Geometry check sheet. Reference: the model listing, model coordinates, mm. Face numbers are marked on the shaded views. Coordinates: 2 decimals unless noted, no trailing zeros. Loops run counter-clockwise (first coordinate to the right, second up) from the corner with the lowest first, then second, coordinate; pieces in that order, holes last.
from build123d import *

# Parameters (mm, degrees)
SKETCH1_W                            = 90
SKETCH1_H                            = 120
BOSS_EXTRUDE2_DEPTH                  = 4
SKETCH5_W                            = 12.2
SKETCH5_H                            = 22.5
CUT_EXTRUDE1_DEPTH                   = 76.106590923
BOSS_EXTRUDE4_START                  = 45
SKETCH10_W                           = 30.35
SKETCH10_H                           = 30.35
SKETCH10_R                           = 7.75
BOSS_EXTRUDE4_DEPTH                  = 25
BOSS_EXTRUDE5_START                  = -20
SKETCH10_4_W                         = 30.35
SKETCH10_4_H                         = 30.35
SKETCH10_4_R                         = 7.75
BOSS_EXTRUDE5_DEPTH                  = 25
CHAMFER6_SIZE                        = 5
CHAMFER7_SIZE                        = 10
F_3_0_3_DIAMETER_HOLE2_D             = 3
MIRROR9_AT_THE_SECOND_PLANE_COPY_1_D = 3
F_3_0_3_DIAMETER_HOLE3_D             = 3


with BuildPart() as part:
    # Sketch1 → Boss-Extrude2 (new body)
    with BuildSketch(Plane(origin=(0, 0, 0), x_dir=(1, 0, 0), z_dir=(0, 1, 0))):
        Rectangle(SKETCH1_W, SKETCH1_H)
    extrude(amount=BOSS_EXTRUDE2_DEPTH)

    # Sketch5 → Cut-Extrude1 (cut, through all)
    with BuildSketch(Plane(origin=(0, 4, 0), x_dir=(1, 0, 0), z_dir=(0, 1, 0))):
        with Locations((-23.9, 33.75)):
            Rectangle(SKETCH5_W, SKETCH5_H)
        with Locations((23.9, 33.75)):
            Rectangle(SKETCH5_W, SKETCH5_H)
    extrude(amount=-CUT_EXTRUDE1_DEPTH, mode=Mode.SUBTRACT)

    # Sketch10 → Boss-Extrude4 (add)
    # profile 1 of 3: a face of its own
    with BuildSketch(Plane(origin=(0, 0, 0), x_dir=(0, 0, -1), z_dir=(1, 0, 0)).offset(BOSS_EXTRUDE4_START)):
        with Locations((-29.825, 19.175)):
            Rectangle(SKETCH10_W, SKETCH10_H)
        with Locations((-29.825, 19.175)):
            Circle(SKETCH10_R, mode=Mode.SUBTRACT)
    # profile 2 of 3: a face of its own
    with BuildSketch(Plane(origin=(0, 0, 0), x_dir=(0, 0, -1), z_dir=(1, 0, 0)).offset(BOSS_EXTRUDE4_START)):
        with BuildLine():
            ThreePointArc((-25.604514246, 25.675), (-29.825, 26.925), (-34.045485754, 25.675))
            Line((-34.045485754, 25.675), (-25.604514246, 25.675))
        make_face()
    # profile 3 of 3: a face of its own
    with BuildSketch(Plane(origin=(0, 0, 0), x_dir=(0, 0, -1), z_dir=(1, 0, 0)).offset(BOSS_EXTRUDE4_START)):
        with BuildLine():
            Line((-25.604514246, 12.675), (-34.045485754, 12.675))
            ThreePointArc((-34.045485754, 12.675), (-29.825, 11.425), (-25.604514246, 12.675))
        make_face()
    extrude(amount=-BOSS_EXTRUDE4_DEPTH)

    # Sketch10<4> → Boss-Extrude5 (add)
    # profile 1 of 3: a face of its own
    with BuildSketch(Plane(origin=(0, 0, 0), x_dir=(0, 0, -1), z_dir=(1, 0, 0)).offset(BOSS_EXTRUDE5_START)):
        with Locations((-29.825, 19.175)):
            Rectangle(SKETCH10_4_W, SKETCH10_4_H)
        with Locations((-29.825, 19.175)):
            Circle(SKETCH10_4_R, mode=Mode.SUBTRACT)
    # profile 2 of 3: a face of its own
    with BuildSketch(Plane(origin=(0, 0, 0), x_dir=(0, 0, -1), z_dir=(1, 0, 0)).offset(BOSS_EXTRUDE5_START)):
        with BuildLine():
            ThreePointArc((-25.604514246, 25.675), (-29.825, 26.925), (-34.045485754, 25.675))
            Line((-34.045485754, 25.675), (-25.604514246, 25.675))
        make_face()
    # profile 3 of 3: a face of its own
    with BuildSketch(Plane(origin=(0, 0, 0), x_dir=(0, 0, -1), z_dir=(1, 0, 0)).offset(BOSS_EXTRUDE5_START)):
        with BuildLine():
            Line((-25.604514246, 12.675), (-34.045485754, 12.675))
            ThreePointArc((-34.045485754, 12.675), (-29.825, 11.425), (-25.604514246, 12.675))
        make_face()
    extrude(amount=-BOSS_EXTRUDE5_DEPTH)

    # Chamfer6
    chamfer6_edges = [part.edges().sort_by_distance(p)[0] for p in [
        (-45, 2, 60),
        (-45, 2, -60),
        (45, 2, -60),
        (45, 2, 60),
    ]]
    chamfer(chamfer6_edges, length=CHAMFER6_SIZE)

    # Chamfer7
    chamfer7_edges = [part.edges().sort_by_distance(p)[0] for p in [
        (32.5, 4, 45),
        (32.5, 34.35, 45),
        (32.5, 34.35, 14.65),
        (32.5, 4, 14.65),
        (-32.5, 34.35, 45),
        (-32.5, 4, 45),
        (-32.5, 4, 14.65),
        (-32.5, 34.35, 14.65),
    ]]
    chamfer(chamfer7_edges, length=CHAMFER7_SIZE)

    # Ø3.0 (3) Diameter Hole2 (through all)
    with Locations(Plane.XZ):
        with Locations((-35.428932188, 50.428932188)):
            f_3_0_3_diameter_hole2 = Hole(F_3_0_3_DIAMETER_HOLE2_D / 2)

    # Mirror9: Ø3.0 (3) Diameter Hole2 across plane
    add(f_3_0_3_diameter_hole2.mirror(Plane.XY), mode=Mode.SUBTRACT)

    # Mirror9 at the second plane: Ø3.0 (3) Diameter Hole2 across plane
    add(f_3_0_3_diameter_hole2.mirror(Plane(origin=(0, 0, 0), x_dir=(0, 0, 1), z_dir=(1, 0, 0))), mode=Mode.SUBTRACT)

    # Mirror9 at the second plane copy 1 (through all)
    with Locations(Plane(origin=(0, 0, 0), x_dir=(-1, 0, 0), z_dir=(0, -1, 0))):
        with Locations((-35.428932188, 50.428932188)):
            Hole(MIRROR9_AT_THE_SECOND_PLANE_COPY_1_D / 2)

    # Ø3.0 (3) Diameter Hole3 (through all)
    with Locations(Plane.XZ):
        with Locations((-23.9, -19.85), (-23.9, -47.65)):
            f_3_0_3_diameter_hole3 = Hole(F_3_0_3_DIAMETER_HOLE3_D / 2)

    # Mirror10: Ø3.0 (3) Diameter Hole3 across plane
    add(f_3_0_3_diameter_hole3.mirror(Plane(origin=(0, 0, 0), x_dir=(0, 0, 1), z_dir=(1, 0, 0))), mode=Mode.SUBTRACT)


solid = part.part
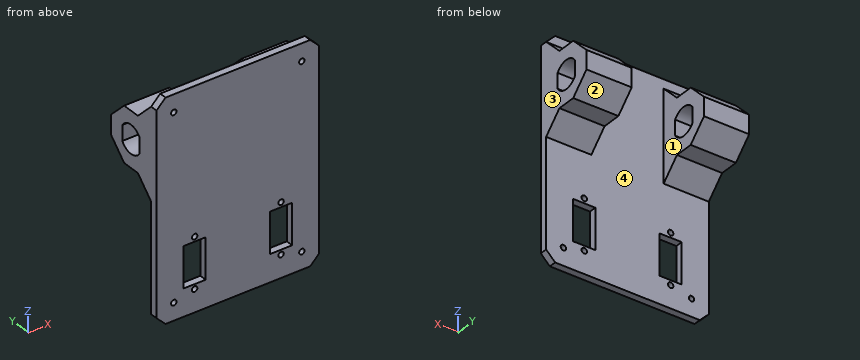
(1) Draft check along X on the marked faces 1, 2, 3 and 4. Enter one of: +X half, -X half, draft (parallel to the pull), parting line (faces both ways), or undercut.
Findings:
face 1: undercut
face 2: draft
face 3: +X half
face 4: undercut
(2) Sectioned sample at A-A on z = -47.65. Record the cut outline in (x, y), and give its area (3 significant figures).
Findings:
outline: (-45, 0) - (-25.4, 0) - (-25.4, 4) - (-45, 4) - close; (-22.4, 0) - (22.4, 0) - (22.4, 4) - (-22.4, 4) - close; (25.4, 0) - (45, 0) - (45, 4) - (25.4, 4) - close
area: 336 mm2
(3) Scan lines: L1, parallel to Z at x = -23.9, y = 2.3; L2, parallel to X at y = 10, z = 32.5; L3, parallel to Y at x = -29, z = 32 (3 decimals). Record each from-to range of solid material in increasing order.
Findings:
L1: z = -60 to -49.15, -46.15 to -45, -22.5 to -21.35, -18.35 to 60
L2: x = -45 to -20, 20 to 45
L3: y = 0 to 12.675, 25.675 to 34.35
(4) Gauge pin test, flat ends, axial feed: pin 1 Ø3 at (x, y) = (-38.5, 20.5) entering from -Z; pin 2 Ø4 at (x, z) = (35.43, -50.43) entering from -Y; pin 3 Ø5 at (x, z) = (4, 37) entering from +Y; pin 4 Ø3 at (x, y) = (-34.5, 20.5) entering from +Z. Record the tip position at first contact, or that the pin passes through.
Findings:
pin 1: stops at z = 14.65
pin 2: stops at y = 0
pin 3: stops at y = 4
pin 4: stops at z = 45
(5) Sectioned sample at C-C on y = 29. Record the cut outline in (x, z), and give its area (3 significant figures).
Findings:
outline: (-45, 19.3) - (-20, 19.3) - (-20, 40.35) - (-45, 40.35) - close; (20, 19.3) - (45, 19.3) - (45, 40.35) - (20, 40.35) - close
area: 1,050 mm2
(6) Sectioned sample at D-D on y = 7. Record the cut outline in (x, z), and give its area (3 significant figures).
Findings:
outline: (-45, 7.65) - (-20, 7.65) - (-20, 52) - (-45, 52) - close; (20, 7.65) - (45, 7.65) - (45, 52) - (20, 52) - close; hole circle Ø3 at (-35.43, 50.43); hole circle Ø3 at (35.43, 50.43)
area: 2,200 mm2
(7) Sectioned sample at B-B on x = 23.9. Record the cut outline in (y, z) (3 decimals), and give its area (3 significant figures).
Findings:
outline: (0, -60) - (4, -60) - (4, -49.15) - (0, -49.15) - close; (0, -46.15) - (4, -46.15) - (4, -45) - (0, -45) - close; (0, -22.5) - (4, -22.5) - (4, -21.35) - (0, -21.35) - close; (0, -18.35) - (4, -18.35) - (4, 4.65) - (14, 14.65) - (24.35, 14.65) - (34.35, 24.65) - (34.35, 35) - (24.35, 45) - (14, 45) - (4, 55) - (4, 60) - (0, 60) - close; hole (12.675, 25.605) arc R7.75 ccw to (25.675, 25.605) - (25.675, 34.045) arc R7.75 ccw to (12.675, 34.045) - close
area: 1,110 mm2
